Source: CAD feature listing. Evaluate the final solid. Frame: model axes, mm. A direction names the side the tool comes from. Round coordinates to 2 decimals unless told otherwise and drop trailing zeros. Loops run counter-clockwise (first coordinate to the right, second up) from the corner with the lowest first, then second, coordinate; pieces in that order, holes last. Notation, with made-up numbers: (-32.5, 50.5) - (4.5, 50.5) arc R16 cw to (4.5, 79.5) - close; hole circle Ø2 at (35.5, 29). An arc over 180 degrees is marked (long way). One line per question, with ' | ' between items.
from build123d import *

# Parameters (mm, degrees)
EXTRUDE_1_DEPTH     = 120
SKETCH_2_R          = 1.5
CUT_EXTRUDE_1_DEPTH = 124.490890352
SKETCH_3_R          = 1.5
CUT_EXTRUDE_2_DEPTH = 124.803271362


with BuildPart() as part:
    # 草图1 → 凸台-拉伸1 (new body)
    with BuildSketch(Plane.XY):
        Polygon((0, 0), (26.5, 0), (26.5, -1.5), (1.5, -1.5), (1.5, -15), (0, -15), align=None)
    extrude(amount=EXTRUDE_1_DEPTH)

    # 草图2 → 切除-拉伸1 (cut, through all)
    with BuildSketch(Plane(origin=(1.5, 0, 0), x_dir=(0, 0, -1), z_dir=(1, 0, 0))):
        with Locations(Location((-60, -7.5, 0), (0, 0, 90))):
            Circle(SKETCH_2_R)
        with Locations(Location((-107, -7.5, 0), (0, 0, 90))):
            Circle(SKETCH_2_R)
        with Locations(Location((-13, -7.5, 0), (0, 0, 90))):
            Circle(SKETCH_2_R)
    extrude(amount=-CUT_EXTRUDE_1_DEPTH, mode=Mode.SUBTRACT)

    # 草图3 → 切除-拉伸2 (cut, through all)
    with BuildSketch(Plane(origin=(0, 0, 0), x_dir=(1, 0, 0), z_dir=(0, 1, 0))):
        with Locations(Location((6, -107.5, 0), (0, 0, 270))):
            Circle(SKETCH_3_R)
        with Locations(Location((6, -12.5, 0), (0, 0, 270))):
            Circle(SKETCH_3_R)
    extrude(amount=-CUT_EXTRUDE_2_DEPTH, mode=Mode.SUBTRACT)


solid = part.part
1. Section query A-A, the plane x = 6. Return loops of the section in (y, z).
Worked out:
outline: (-1.5, 0) - (0, 0) - (0, 11) - (-1.5, 11) - close; (-1.5, 14) - (0, 14) - (0, 106) - (-1.5, 106) - close; (-1.5, 109) - (0, 109) - (0, 120) - (-1.5, 120) - close
2. Section query C-C, the plane z = 13. Return loops of the section in (x, y).
Worked out:
outline: (0, -15) - (1.5, -15) - (1.5, -9) - (0, -9) - close; (0, -6) - (1.5, -6) - (1.5, -1.5) - (4.59, -1.5) - (4.59, 0) - (0, 0) - close; (7.41, -1.5) - (26.5, -1.5) - (26.5, 0) - (7.41, 0) - close
3. Section query D-D, the plane z = 35.5. Return loops of the section in (x, y).
Worked out:
outline: (0, -15) - (1.5, -15) - (1.5, -1.5) - (26.5, -1.5) - (26.5, 0) - (0, 0) - close
4. Material intervals for probe 1 along Z at (x, y) = (0.65, -7.5); probe 2 along Y at (x, z) = (2.75, 104); probe 3 along X at (y, z) = (-2.5, 88), sorted ascending.
Worked out:
probe 1: z = 0 to 11.5, 14.5 to 58.5, 61.5 to 105.5, 108.5 to 120 | probe 2: y = -1.5 to 0 | probe 3: x = 0 to 1.5
5. Access query for faces 1 (the flat face through (14, -1.5, 59)), 2 (the cylindrical face through (0.76, -7.695, 108.487)). Directions: +Z, -Z, +X, -X, +Y, -Y. A direction counts if a zero-diameter tool reaches every point of the face in a straight line with its end or side. Return the directions, or none.
Worked out:
face 1: +Z, -Z, +X, -Y | face 2: +X, -X
6. Contact query for flat-ended pins moving along their axis: P1, Ø7.5, axis at x = 12, z = 62.5, coming from the -Y side; P2, Ø3, axis at x = 6.5, z = 86, coming from the +Y side; P3, Ø1.8, axis at y = -7.5, z = 60, coming from the -X side; P4, Ø3, axis at y = -10.5, z = 28.5, coming from the +X side. Output: stop coordinate, or through.
Worked out:
P1: stops at y = -1.5 | P2: stops at y = 0 | P3: passes through | P4: stops at x = 1.5
7. Mould query, pull axis X, two halves, no side actions, for faces 3 (the flat face through (1.5, -10, 59)), 4 (the cylindrical face through (6, -1, 106)), 5 (the flat face through (11, -1, 120)). Classes: released by +X, released by -X, zero draft, split by the parting line, or undercut.
Worked out:
face 3: released by +X | face 4: undercut | face 5: zero draft
8. Section query B-B, the plane y = -7.5. Return loops of the section in (x, z), plus the area to 4 significant figures.
Worked out:
outline: (0, 0) - (1.5, 0) - (1.5, 11.5) - (0, 11.5) - close; (0, 14.5) - (1.5, 14.5) - (1.5, 58.5) - (0, 58.5) - close; (0, 61.5) - (1.5, 61.5) - (1.5, 105.5) - (0, 105.5) - close; (0, 108.5) - (1.5, 108.5) - (1.5, 120) - (0, 120) - close | area: 166.5 mm2
